Model file for the job. Use its own axes, mm. A direction names the side the tool comes from. Give positions to 0.01 mm unless a question says otherwise; leave off trailing zeros. Order: outer loops, then holes, each group sorted by start corner. A loop starts at its lowest first (then second) coordinate and runs counter-clockwise, first axis right, second up. Notation, with made-up numbers: M -0.5,0 L 24.5,0 A22 ccw 24.5,26 Z; hole C -37,73 d5. An arc over 180 degrees is marked long. Return JSON: item names as keys, results as strings. Group by question number.
1. Wall check: probe 1 along X at (y, z) = (14.5, 2.25); probe 2 along Y at (x, z) = (-8, 3.5). Give the ranges that are in metal, low to high. Write a range as [from, to].
2. Slice it at A-A on x = -18.25. List the corners of the cut face in (y, z), then the cut area to 3 significant figures.
3. 3-axis set-ups, long thin cutter, end or side, ignore diameter. For faces 1 (the face through (-5, 15, 3)), 2 (the face through (-3, 5, 15)), 3 (the face through (-15, 3, 5)): which of +Z, -Z, +X, -X, +Y, -Y reach the whole face in a straight line?
4. Pin check, flat tips, straight feed: pin 1 (10 mm diameter, centred on y = 9, z = 22, fed in from +X); pin 2 (1.5 mm diameter, centred on x = -12.5, y = 3.5, fed in from +Z); pin 3 (10 mm diameter, centred on x = -13, z = 4.5, fed in from +Y); pin 4 (5.5 mm diameter, centred on y = 1.5, z = 16, fed in from -X). Stop position of each tip, or through.
5. Slice it at C-C on z = 15. List the corners of the cut face in (x, y).
6. Slice it at B-B on y = 7.5. List the corners of the cut face in (x, z).
7. Slice it at D-D on x = -3.25. List the corners of the cut face in (y, z), then the cut area to 3 significant figures.
from build123d import *

# Parameters (mm, degrees)
F1_DEPTH = 5
F2_W     = 5
F2_H     = 5
F3_DEPTH = 20
F4_SIZE  = 1


with BuildPart() as f1:
    # F0 (on Top) → F1 (new body)
    with BuildSketch(Plane.XY):
        Polygon((-25, 0), (0, 0), (0, 25), (-5, 25), (-5, 5), (-25, 5), align=None)
    extrude(amount=F1_DEPTH)

    # F2 (on face) → F3 (join)
    with BuildSketch(Plane.XY.offset(5)):
        with Locations((-2.5, 2.5)):
            Rectangle(F2_W, F2_H)
    extrude(amount=F3_DEPTH)

    # F4
    f4_edges = [f1.edges().sort_by_distance(p)[0] for p in [
        (-12.5, 0, 0),
        (0, 12.5, 0),
        (-2.5, 25, 0),
        (-5, 15, 0),
        (-15, 5, 0),
        (-25, 2.5, 0),
    ]]
    chamfer(f4_edges, length=F4_SIZE)


solid = f1.part
Result:
{
 "1": {"probe 1": "x = [-5, 0]", "probe 2": "y = [0, 5]"},
 "2": {"outline": "M 0,1 L 1,0 L 4,0 L 5,1 L 5,5 L 0,5 Z", "area": "24.0 mm2"},
 "3": {"face 1": "+Z, -Z, -X, +Y", "face 2": "+Z, +X, -X, +Y", "face 3": "+Z, -X, +Y, -Y"},
 "4": {"pin 1": "stops at x = 0", "pin 2": "stops at z = 5", "pin 3": "stops at y = 5", "pin 4": "stops at x = -5"},
 "5": {"outline": "M -5,0 L 0,0 L 0,5 L -5,5 Z"},
 "6": {"outline": "M -5,1 L -4,0 L -1,0 L 0,1 L 0,5 L -5,5 Z"},
 "7": {"outline": "M 0,1 L 1,0 L 24,0 L 25,1 L 25,5 L 5,5 L 5,25 L 0,25 Z", "area": "224 mm2"}
}
